Read the model definition and answer for the solid it produces. Units are mm, in the model's axes. A direction names the side the tool comes from. Coordinates: 2 decimals unless noted, no trailing zeros. Write each loop counter-clockwise with the first axis right and the second up, starting at its lowest first coordinate (ties: lowest second). Pieces come first, ordered by that corner, then holes. Notation, with made-up numbers: (-4, 66) - (20, 66) arc R29 cw to (20, 97) - close; hole circle Ø7 at (-14, -15.5). An arc over 180 degrees is marked (long way). Return JSON: item names as keys, results as strings.
```python
from build123d import *

# Parameters (mm, degrees)
SKICA1_W                 = 100
SKICA1_H                 = 80
P_IDAT_VYSUNUT_M1_DEPTH  = 3
ODEBRAT_START            = -0.4
SKICA2_R                 = 3
ODEBRAT_VYSUNUT_M1_DEPTH = 1.4


with BuildPart() as part:
    # Skica1 → Přidat vysunutím1 (new body)
    with BuildSketch(Plane.XY):
        with Locations((50, 40)):
            Rectangle(SKICA1_W, SKICA1_H)
    extrude(amount=P_IDAT_VYSUNUT_M1_DEPTH)

    # Skica2 → Odebrat vysunutím1 (cut)
    with BuildSketch(Plane.XY.offset(3).offset(ODEBRAT_START)):
        with Locations((4, 76)):
            Circle(SKICA2_R)
        with Locations((96, 76)):
            Circle(SKICA2_R)
        with Locations((96, 4)):
            Circle(SKICA2_R)
        with Locations((4, 4)):
            Circle(SKICA2_R)
    extrude(amount=-ODEBRAT_VYSUNUT_M1_DEPTH, mode=Mode.SUBTRACT)


solid = part.part
```
(1) Which of the six approach directions +Z, -Z, +X, -X, +Y, -Y give full straight-line access (tool end or side, diameter ignored) to faces 4 (the face through (93.6, 74.2, 1.9)), 5 (the face through (49, 41, 3))?
Answer:
{"face 4": "none", "face 5": "+Z, +X, -X, +Y, -Y"}
(2) A straight line is drawn through the part: line 1 (Y direction, x = 96, z = 1.6). Find the intervals that lie inside material, in ascending order. Write a range as from..to.
Answer:
{"line 1": "0..1, 7..73, 79..80"}
(3) A cutting plane is placed at A-A (y = 76). Determine the outline of the cut face in (x, z), and give its area (3 significant figures).
Answer:
{"outline": "(0, 0) - (100, 0) - (100, 3) - (0, 3) - close; hole (1, 1.2) - (7, 1.2) - (7, 2.6) - (1, 2.6) - close; hole (93, 1.2) - (99, 1.2) - (99, 2.6) - (93, 2.6) - close", "area": "283 mm²"}
(4) Determine the mould class of faces 1 (the face through (3.35, 73.07, 1.91)), 2 (the face through (100, 39, 1)), 3 (the face through (49, 80, 1)) for opening direction X: +X half, -X half, draft (parallel to the pull), parting line (faces both ways), or undercut.
Answer:
{"face 1": "undercut", "face 2": "+X half", "face 3": "draft"}
(5) A cutting plane is placed at B-B (x = 96). Determine the outline of the cut face in (y, z).
Answer:
{"outline": "(0, 0) - (80, 0) - (80, 3) - (0, 3) - close; hole (1, 1.2) - (7, 1.2) - (7, 2.6) - (1, 2.6) - close; hole (73, 1.2) - (79, 1.2) - (79, 2.6) - (73, 2.6) - close"}
